Here's the drawing with two shaded views (mm, measured from the low corner). I have some questions. A direction names the side the tool comes from. Coordinates: 2 decimals unless noted, no trailing zeros. Loops run counter-clockwise (first coordinate to the right, second up) from the corner with the lowest first, then second, coordinate; pieces in that order, holes last. Notation, with made-up numbers: (44.5, 23) - (68.5, 23) arc R12 ccw to (68.5, 45) - close; hole circle Ø8 at (56, -11.75). An arc over 180 degrees is marked (long way). One line per item, written item: value. Start each with the question number.
(1) If we section it at A-A on z = 11.5: Write out the boundary of the cut face in (x, y) (3 decimals).
(2) If we section it at C-C on z = 4.5: Write out the boundary of the cut face in (x, y).
(3) If I drill on line 1 along X through (y, z) = (7.5, 11.5) (3 decimals); line 2 along Z through (x, y) = (6, 7); line 3 along X through (y, z) = (4, 15.5), over which ranges is the centre line in solid material (lowest first)? Write a range as from..to.
(4) If we section it at D-D on y = 26: Write out the boundary of the cut face in (x, z) (3 decimals), then the cut area to 3 significant figures.
(5) If we section it at B-B on x = 11.5: Write out the boundary of the cut face in (y, z) (3 decimals), then the cut area to 4 significant figures.
(6) I'm going to push flat-ended pins straight in: P1, Ø12, axis at x = 6, y = 20.5, coming from the -Z side (3 decimals); P2, Ø0.9, axis at x = 2, y = 13.5, coming from the +Z side; P3, Ø0.6, axis at x = 2.5, y = 10, coming from the -Z side; P4, Ø5, axis at x = 11.5, z = 19.5, coming from the -Y side. Where does each tip first touch, or does it pass through?
(7) On a 3-axis mill with a long thin cutter (end or side, diameter ignored), from which of +Z, -Z, +X, -X, +Y, -Y can I reach the whole of each face in a straight line? I mean the marked faces 1 and 2. Say none if no direction works.
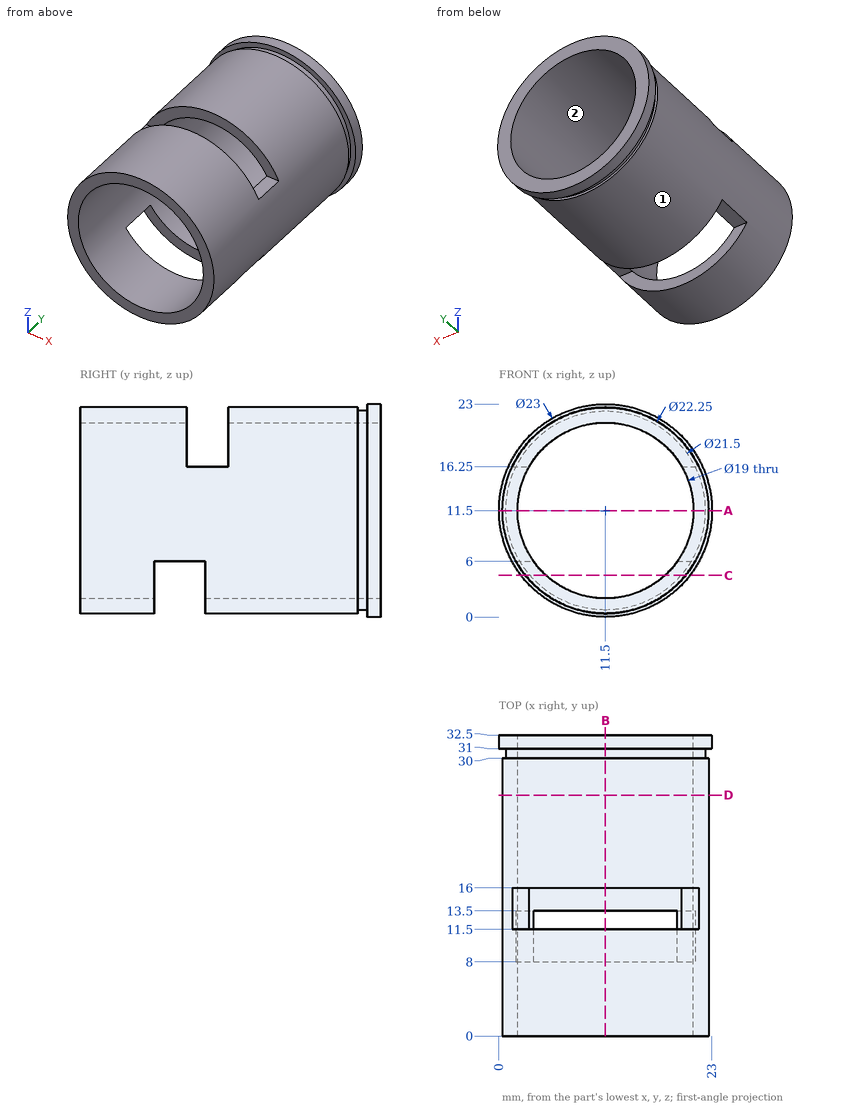
Values:
1. outline: (0, 31) - (0.75, 31) - (0.75, 30) - (0.375, 30) - (0.375, 0) - (2, 0) - (2, 32.5) - (0, 32.5) - close; (21, 0) - (22.625, 0) - (22.625, 30) - (22.25, 30) - (22.25, 31) - (23, 31) - (23, 32.5) - (21, 32.5) - close
2. outline: (2.38, 31) - (3.34, 31) - (3.34, 30) - (2.85, 30) - (2.85, 13.5) - (5.08, 13.5) - (5.08, 32.5) - (2.38, 32.5) - close; (2.85, 0) - (5.08, 0) - (5.08, 8) - (2.85, 8) - close; (17.92, 0) - (20.15, 0) - (20.15, 8) - (17.92, 8) - close; (17.92, 13.5) - (20.15, 13.5) - (20.15, 30) - (19.66, 30) - (19.66, 31) - (20.62, 31) - (20.62, 32.5) - (17.92, 32.5) - close
3. line 1: x = 0.375..2, 21..22.625
3. line 2: z = 1.83..3.75, 19.25..21.17
3. line 3: x = 1.12..2.88, 20.12..21.88
4. outline: circle Ø22.25 at (11.5, 11.5); hole circle Ø19 at (11.5, 11.5)
4. area: 105 mm2
5. outline: (0, 0.375) - (8, 0.375) - (8, 2) - (0, 2) - close; (0, 21) - (11.5, 21) - (11.5, 22.625) - (0, 22.625) - close; (13.5, 0.375) - (30, 0.375) - (30, 0.75) - (31, 0.75) - (31, 0) - (32.5, 0) - (32.5, 2) - (13.5, 2) - close; (16, 21) - (32.5, 21) - (32.5, 23) - (31, 23) - (31, 22.25) - (30, 22.25) - (30, 22.625) - (16, 22.625) - close
5. area: 89.75 mm2
6. P1: stops at z = 0.375
6. P2: stops at z = 16.25
6. P3: stops at z = 6
6. P4: stops at y = 0
7. face 1: -Y
7. face 2: +Y, -Y
